from build123d import *

# Parameters (mm, degrees)
ESQUISSE1_R        = 7.9
BOSS_EXTRU_1_DEPTH = 1.4


with BuildPart() as part:
    # Esquisse1 → Boss.-Extru.1 (new body, symmetric)
    with BuildSketch(Plane.XY):
        Polygon((10.854185061, 0), (5.42709253, 9.4), (-5.42709253, 9.4), (-10.854185061, 0), (-5.42709253, -9.4), (5.42709253, -9.4), align=None)
        Circle(ESQUISSE1_R, mode=Mode.SUBTRACT)
    extrude(amount=BOSS_EXTRU_1_DEPTH, both=True)

    # Esquisse2 → Enlèvement de matière-Révolution1 (revolve, cut)
    with BuildSketch(Plane(origin=(0, 0, 0), x_dir=(1, 0, 0), z_dir=(0, 1, 0))):
        with BuildLine():
            Line((-10.854185061, 1.4), (-10.854185061, 0.4))
            ThreePointArc((-10.854185061, 0.4), (-9.866861873, 0.925353624), (-8.854185061, 1.4))
            Line((-8.854185061, 1.4), (-10.854185061, 1.4))
        make_face()
    enl_vement_de_mati_re_r_volution1 = revolve(axis=Axis((0, 0, 0), (0, 0, -1)), mode=Mode.SUBTRACT)

    # Symétrie1: Enlèvement de matière-Révolution1 across plane
    add(enl_vement_de_mati_re_r_volution1.mirror(Plane.XY), mode=Mode.SUBTRACT)


solid = part.part
Geometry check sheet. Reference: the model listing, model coordinates, mm. Coordinates: 2 decimals unless noted, no trailing zeros. Answer in a Markdown table with one row per item. Add a question column.
1) Release check for a two-part mould opening along X. For faces 1 (the flat face through (-8.2, -4.6, 0)), 2 (the flat face through (8.2, 4.6, 0)), 3 (the cylindrical face through (-6.269, -4.807, -0.02)), 4 (the flat face through (-8, -1, -1.4)) record: +X half, -X half, draft (parallel to the pull), parting line (faces both ways), or undercut.
2) Gauge pin test, flat ends, axial feed: P1, Ø3, axis at x = 4.5, y = 1, coming from the -Z side; P2, Ø1.5, axis at y = -3, z = -1, coming from the +X side. Record the tip position at first contact, or that the pin passes through.
3) Material ranges on line 1 along Y through (x, z) = (0, 0.7); line 2 along X through (y, z) = (-6, -0.8); line 3 along X through (y, z) = (2.75, 1.1), recorded low to high. Write a range as [from, to].
Check result:
| question | item | result |
|---|---|---|
| 1 | face 1 | -X half |
| 1 | face 2 | +X half |
| 1 | face 3 | undercut |
| 1 | face 4 | draft |
| 2 | P1 | passes through |
| 2 | P2 | stops at x = 9.55 |
| 3 | line 1 | y = [-9.4, -7.9], [7.9, 9.4] |
| 3 | line 2 | x = [-7.39, -5.14], [5.14, 7.39] |
| 3 | line 3 | x = [-9.1, -7.41], [7.41, 9.1] |
